```python
from build123d import *

# Parameters (mm, degrees)
BOSS_EXTRUDE3_DEPTH = 3
BOSS_EXTRUDE4_DEPTH = 1.5
FILLET1_R           = 0.2


with BuildPart() as part:
    # Sketch3 → Boss-Extrude3 (new body)
    with BuildSketch(Plane.XY):
        with BuildLine():
            Line((-25.35426057, 19.199439056), (-25.35426057, -14.681488353))
            ThreePointArc((-25.35426057, -14.681488353), (-24.197332356, -17.474560138), (-21.40426057, -18.631488353))
            Line((-21.40426057, -18.631488353), (18.774241414, -18.631488353))
            ThreePointArc((18.774241414, -18.631488353), (21.567313199, -17.474560138), (22.724241414, -14.681488353))
            Line((22.724241414, -14.681488353), (22.724241414, 19.199439056))
            ThreePointArc((22.724241414, 19.199439056), (21.567313199, 21.992510842), (18.774241414, 23.149439056))
            Line((18.774241414, 23.149439056), (-21.40426057, 23.149439056))
            ThreePointArc((-21.40426057, 23.149439056), (-24.197332356, 21.992510842), (-25.35426057, 19.199439056))
        make_face()
    extrude(amount=BOSS_EXTRUDE3_DEPTH)

    # Sketch3<4> → Boss-Extrude4 (add)
    with BuildSketch(Plane.XY):
        with BuildLine():
            Line((-27.40426057, 19.199439056), (-27.40426057, -14.681488353))
            ThreePointArc((-27.40426057, -14.681488353), (-25.646901258, -18.92412904), (-21.40426057, -20.681488353))
            Line((-21.40426057, -20.681488353), (18.774241414, -20.681488353))
            ThreePointArc((18.774241414, -20.681488353), (23.016882101, -18.92412904), (24.774241414, -14.681488353))
            Line((24.774241414, -14.681488353), (24.774241414, 19.199439056))
            ThreePointArc((24.774241414, 19.199439056), (23.016882101, 23.442079743), (18.774241414, 25.199439056))
            Line((18.774241414, 25.199439056), (-21.40426057, 25.199439056))
            ThreePointArc((-21.40426057, 25.199439056), (-25.646901258, 23.442079743), (-27.40426057, 19.199439056))
        make_face()
        with BuildLine():
            Line((-25.35426057, 19.199439056), (-25.35426057, -14.681488353))
            ThreePointArc((-25.35426057, -14.681488353), (-24.197332356, -17.474560138), (-21.40426057, -18.631488353))
            Line((-21.40426057, -18.631488353), (18.774241414, -18.631488353))
            ThreePointArc((18.774241414, -18.631488353), (21.567313199, -17.474560138), (22.724241414, -14.681488353))
            Line((22.724241414, -14.681488353), (22.724241414, 19.199439056))
            ThreePointArc((22.724241414, 19.199439056), (21.567313199, 21.992510842), (18.774241414, 23.149439056))
            Line((18.774241414, 23.149439056), (-21.40426057, 23.149439056))
            ThreePointArc((-21.40426057, 23.149439056), (-24.197332356, 21.992510842), (-25.35426057, 19.199439056))
        make_face(mode=Mode.SUBTRACT)
    extrude(amount=BOSS_EXTRUDE4_DEPTH)

    # Fillet1
    fillet1_edges = [part.edges().sort_by_distance(p)[0] for p in [
        (-25.646901258, -18.92412904, 0),
        (-1.315009578, -20.681488353, 0),
        (23.016882101, -18.92412904, 0),
        (24.774241414, 2.258975352, 0),
        (23.016882101, 23.442079743, 0),
        (-1.315009578, 25.199439056, 0),
        (-25.646901258, 23.442079743, 0),
        (-27.40426057, 2.258975352, 0),
    ]]
    fillet(fillet1_edges, radius=FILLET1_R)


solid = part.part
```
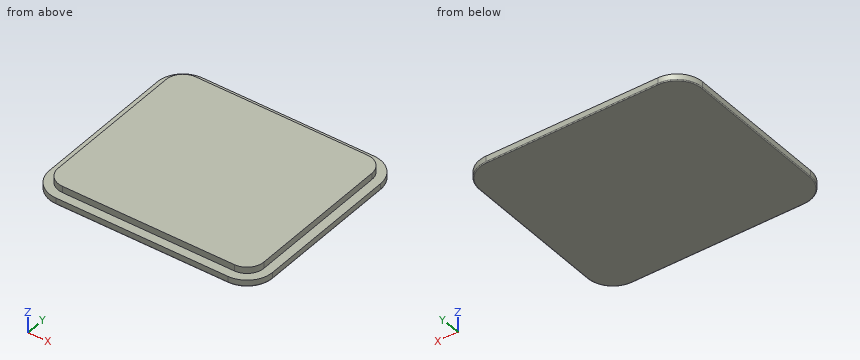
Design review of the part built by this model. Coordinates are the model's own, in mm. Give positions to 0.01 mm unless a question says otherwise; leave off trailing zeros. Order: outer loops, then holes, each group sorted by start corner. A loop starts at its lowest first (then second) coordinate and runs counter-clockwise, first axis right, second up. Notation, with made-up numbers: (-10.5, 30.5) - (23.5, 30.5) arc R21 cw to (23.5, 61.5) - close; hole circle Ø10 at (62.5, 73.5). An arc over 180 degrees is marked (long way). Use a Markdown table: item, result. Add a question column.
(1) Add section A-A on z = 2.5. Give the boundary of the cut face in (x, y), then the cut area to 3 significant figures.
(2) Add section C-C on x = -17.5. Give the boundary of the cut face in (y, z).
(3) Clearance check with flat-ended pins moving along their axes: P1, Ø1.5, axis at x = -19, z = 2, coming from the +Y side; P2, Ø1.6, axis at x = 0, z = 2.5, coming from the +Y side; P3, Ø1.2, axis at y = -5.5, z = 2.5, coming from the +X side; P4, Ø1.6, axis at y = 4.5, z = 2.5, coming from the -X side. State where each tip first meets the part, or that it passes through.
(4) Add section B-B on y = 1.5. Give the boundary of the cut face in (x, z).
(5) Wall thickness on probe 1 along Y at (x, z) = (-13.5, 2.35); probe 2 along X at (y, z) = (17, 2.1); probe 3 along X at (y, z) = (19.5, 0.55): over which ranges is each line inside the solid? List them lowest first. Write a range as [from, to].
Report:
| question | item | result |
|---|---|---|
| 1 | outline | (-25.35, -14.68) arc R3.95 ccw to (-21.4, -18.63) - (18.77, -18.63) arc R3.95 ccw to (22.72, -14.68) - (22.72, 19.2) arc R3.95 ccw to (18.77, 23.15) - (-21.4, 23.15) arc R3.95 ccw to (-25.35, 19.2) - close |
| 1 | area | 2,000 mm² |
| 2 | outline | (-20.68, 0.2) arc R0.2 ccw to (-20.48, 0) - (25, 0) arc R0.2 ccw to (25.2, 0.2) - (25.2, 1.5) - (23.15, 1.5) - (23.15, 3) - (-18.63, 3) - (-18.63, 1.5) - (-20.68, 1.5) - close |
| 3 | P1 | stops at y = 25.2 |
| 3 | P2 | stops at y = 23.15 |
| 3 | P3 | stops at x = 22.72 |
| 3 | P4 | stops at x = -25.35 |
| 4 | outline | (-27.4, 0.2) arc R0.2 ccw to (-27.2, 0) - (24.57, 0) arc R0.2 ccw to (24.77, 0.2) - (24.77, 1.5) - (22.72, 1.5) - (22.72, 3) - (-25.35, 3) - (-25.35, 1.5) - (-27.4, 1.5) - close |
| 5 | probe 1 | y = [-18.63, 23.15] |
| 5 | probe 2 | x = [-25.35, 22.72] |
| 5 | probe 3 | x = [-27.4, 24.77] |
